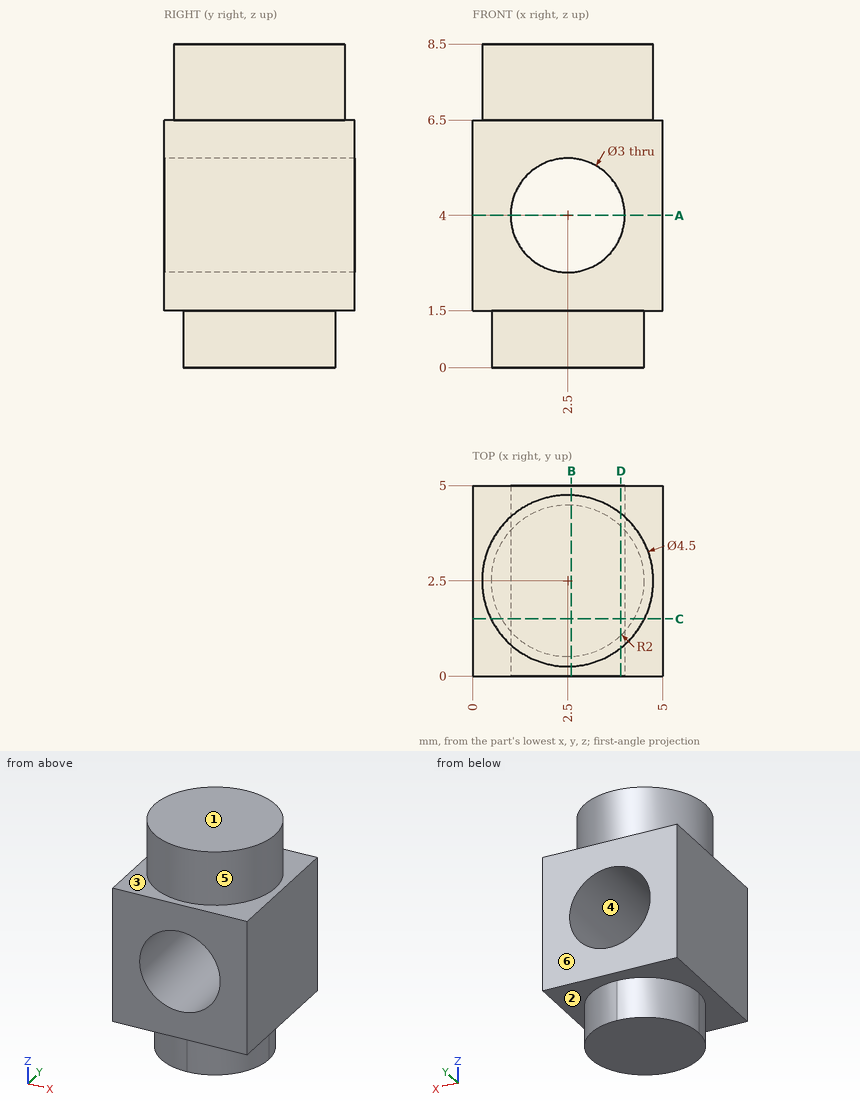
Print and shaded views of the part. All mm, measured from the part's lowest x, y and z. A direction names the side the tool comes from. Give positions to 0.01 mm unless a question says otherwise; leave off trailing zeros. Loops run counter-clockwise (first coordinate to the right, second up) from the corner with the lowest first, then second, coordinate; pieces in that order, holes last. Notation, with made-up numbers: (-38, 5.5) -> (-5, 5.5) arc R17 ccw to (-5, 10.5) -> close; hole circle Ø6 at (75.25, 7). An arc over 180 degrees is marked (long way). One line per question, with ' | ' between items. Start each with the question number.
1) Probe L1, parallel to X at y = 2.7, z = 4; L2, parallel to Z at x = 2.5, y = 1.35; L3, parallel to Z at x = 0.85, y = 4.5. List the from-to ranges inside material, lowest first.
2) 3-axis set-ups, long thin cutter, end or side, ignore diameter. For the marked faces 1, 2 and 3: which of +Z, -Z, +X, -X, +Y, -Y reach the whole face in a straight line?
3) Cut at A-A (z = 4). Give the cut face in (x, y), plus the area to 3 significant figures.
4) Pin check, flat tip, straight feed: pin 1 (1 mm diameter, centred on y = 4, z = 7.5, fed in from +X). Stop position of the tip, or through.
5) Cut at B-B (x = 2.6). Give the cut face in (y, z).
6) Two-plate mould, pull along X, no slides. Class the marked faces 4, 5 and 6: released by +X, released by -X, zero draft, split by the parting line, or undercut.
7) Cut at D-D (x = 3.9). Give the cut face in (y, z).
8) Cut at C-C (y = 1.5). Give the cut face in (x, z), plus the area to 3 significant figures.
Return value:
1) L1: 0 to 1, 4 to 5 | L2: 0 to 2.5, 5.5 to 8.5 | L3: 1.5 to 6.5
2) face 1: +Z, +X, -X, +Y, -Y | face 2: -Z | face 3: +Z
3) outline: (0, 0) -> (1, 0) -> (1, 5) -> (0, 5) -> close; (4, 0) -> (5, 0) -> (5, 5) -> (4, 5) -> close | area: 10.0 mm^2
4) pin 1: x = 4.52
5) outline: (0, 1.5) -> (0.5, 1.5) -> (0.5, 0) -> (4.5, 0) -> (4.5, 1.5) -> (5, 1.5) -> (5, 2.5) -> (0, 2.5) -> close; (0, 5.5) -> (5, 5.5) -> (5, 6.5) -> (4.75, 6.5) -> (4.75, 8.5) -> (0.25, 8.5) -> (0.25, 6.5) -> (0, 6.5) -> close
6) face 4: undercut | face 5: split by the parting line | face 6: zero draft
7) outline: (0, 1.5) -> (1.07, 1.5) -> (1.07, 0) -> (3.93, 0) -> (3.93, 1.5) -> (5, 1.5) -> (5, 3.46) -> (0, 3.46) -> close; (0, 4.54) -> (5, 4.54) -> (5, 6.5) -> (4.26, 6.5) -> (4.26, 8.5) -> (0.74, 8.5) -> (0.74, 6.5) -> (0, 6.5) -> close
8) outline: (0, 1.5) -> (0.77, 1.5) -> (0.77, 0) -> (4.23, 0) -> (4.23, 1.5) -> (5, 1.5) -> (5, 6.5) -> (4.52, 6.5) -> (4.52, 8.5) -> (0.48, 8.5) -> (0.48, 6.5) -> (0, 6.5) -> close; hole circle Ø3 at (2.5, 4) | area: 31.2 mm^2
